Autodesk Inventor part; units mm, degrees
ref_plane "YZ Plane" through (0, 0, 0) normal (1, 0, 0) x (0, 1, 0)
ref_plane "XZ Plane" through (0, 0, 0) normal (0, 1, 0) x (-1, 0, 0)
ref_plane "XY Plane" through (0, 0, 0) normal (0, 0, 1) x (1, 0, 0)
sketch "スケッチ1" plane through (0, 0, 0) normal (0, 0, 1) x (1, 0, 0)
  line L0 (0, 0) -> (10, 0)
  line L1 (10, 0) -> (10, 15)
  line L2 (10, 15) -> (0, 15)
  line L3 (0, 15) -> (0, 0)
  circle A0 centre (5, 15) radius 8.5
  point P0 (0, 8.1261)
  point P1 (10, 8.1261)
  dimension "d0" = 15
  dimension "d1" = 17
  dimension "d27" = 10
  dimension "d28" = 5
extrude "押し出し1" add sketch "スケッチ1" along normal blind 9
sketch "スケッチ2" plane through (0, 0, 9) normal (0, 0, 1) x (1, 0, 0)
  arc A0 (10, 8.1261) -> (0, 8.1261) centre (5, 15) ccw
  point P0 (0, 0)
hole "穴1" at (5, 15, 9) direction (0, 0, -1) diameter 8.3 end through all
sketch "スケッチ3" plane through (0, 0, 9) normal (0, 0, 1) x (1, 0, 0)
  line L0 (0, 0) -> (10, 0)
  line L1 (4.5, 0) -> (5.5, 0)
  line L2 (5.5, 0) -> (5.5, 15)
  line L3 (5.5, 15) -> (4.5, 15)
  line L4 (4.5, 15) -> (4.5, 0)
  line L5 (0, 8.1261) -> (0, 0)
  circle A0 centre (5, 15) radius 4.15
  point P0 (5, 0)
  point P1 (5, 0)
  dimension "d14" = 1
extrude "押し出し2" cut sketch "スケッチ3" against normal up to surface (9 mm away) contours L4 A0 L2 L0 | L4 L3 L2 A0 picked at (4.9443, 13.6178)
sketch "スケッチ4" plane through (10, 0, 0) normal (1, 0, 0) x (0, 0, -1)
  circle A0 centre (-4.5, 4) radius 1.5
  line L0 (0, 0) -> (-9, 0)
  line L1 (0, 0) -> (0, 8.1261)
  line L2 (-4.5, 0) -> (-4.5, 10)
  point P0 (0, 10)
  dimension "d17" = 4
  dimension "d19" = 3
hole "穴2" at (10, 4, 4.5) direction (-1, 0, 0) diameter 4.4 end through all
sketch "スケッチ7" plane through (10, 0, 0) normal (1, 0, 0) x (0, 0, -1)
  circle A0 centre (-4.5, 4) radius 2.2
  line L0 (-4.5, 8.1569) -> (-0.9, 6.0785)
  line L1 (-0.9, 6.0785) -> (-0.9, 1.9215)
  line L2 (-0.9, 1.9215) -> (-4.5, -0.1569)
  line L3 (-4.5, -0.1569) -> (-8.1, 1.9215)
  line L4 (-8.1, 1.9215) -> (-8.1, 6.0785)
  line L5 (-8.1, 6.0785) -> (-4.5, 8.1569)
  line L6 (-9, 10.8802) -> (-9, 0)
  line L7 (0, 0) -> (0, 8.1261)
  line L8 (-9, 10.8802) -> (0, 10.8802)
  line L9 (0, 10.8802) -> (0, 4.0631)
  line L10 (0, 4.0631) -> (-9, 4.0631)
  line L11 (-9, 4.0631) -> (-9, 10.8802)
  point P0 (-4.5, 4)
  point P1 (-0.9, 4.0631)
  point P2 (-8.1, 4.0631)
  dimension "d35" = 7.2
extrude "押し出し5" add sketch "スケッチ7" along normal blind 2 contours L1 L0 L5 L4 L10 L6 L8 L9 L7
chamfer "面取り1" distance 2 angle 45 2 edges at (10, 4.0631, 8.55) (10, 4.0631, 0.45)
equation "\"d28\" = 0.5 * d27"
properties part number "軸止め" material "ABS プラスチック"
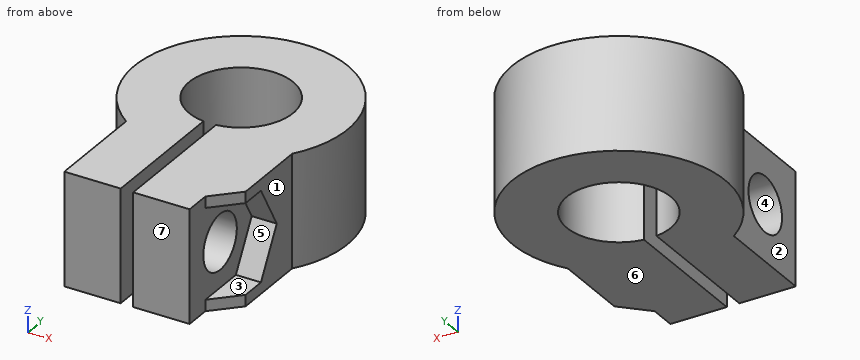
Source: CAD feature listing. Evaluate the final solid. Frame: model axes, mm. Face numbers are marked on the shaded views. A direction names the side the tool comes from. Give positions to 0.01 mm unless a question says otherwise; leave off trailing zeros. Loops run counter-clockwise (first coordinate to the right, second up) from the corner with the lowest first, then second, coordinate; pieces in that order, holes last. Notation, with made-up numbers: M 66,26.25 L 105,26.25 A21 ccw 105,42.25 Z; hole C 33,-17 d1. An arc over 180 degrees is marked long. Put each result on its own line as item: value.
Q1. Section D-D (y = 7.75). Return the cut outline in (x, z).
Response values:
outline: M 0,0 L 4.5,0 L 4.5,9 L 0,9 Z; M 5.5,0 L 12,0 L 12,3.8 L 10,3.8 L 10,5.2 L 12,5.2 L 12,9 L 5.5,9 Z
Q2. Line query: probe 1 along X at (y, z) = (3, 1); probe 2 along Y at (x, z) = (2, 5); probe 3 along Y at (x, z) = (1.9, 4.5). Output: solid intervals per line, ascending. Write a range as [from, to].
Response values:
probe 1: x = [0, 4.5], [5.5, 10]
probe 2: y = [0, 1.86], [6.14, 12.13], [17.87, 22.95]
probe 3: y = [0, 1.8], [6.2, 12.24], [17.76, 22.91]
Q3. Section A-A (y = 15). Return the cut outline in (x, z), and give its area (3 significant figures).
Response values:
outline: M -3.5,0 L 0.85,0 L 0.85,9 L -3.5,9 Z; M 9.15,0 L 13.5,0 L 13.5,9 L 9.15,9 Z
area: 78.3 mm²
Q4. Mould query, pull axis Z, two halves, no side actions, for the marked faces 4, 5, 6 and 7. Classes: released by +Z, released by -Z, zero draft, split by the parting line, or undercut.
Response values:
face 4: undercut
face 5: undercut
face 6: released by -Z
face 7: zero draft
Q5. Section B-B (x = 4.25). Return the cut outline in (y, z).
Response values:
outline: M 0,0 L 10.92,0 L 10.92,9 L 0,9 Z; M 19.08,0 L 23.47,0 L 23.47,9 L 19.08,9 Z; hole C 4,4.5 d4.4
Q6. Reachability of the marked faces 1, 2 and 3 from +Z, -Z, +X, -X, +Y, -Y: full face, straight path, thin tool, end or side. Return the list, or none.
Response values:
face 1: +Z, -Z, +X, -Y
face 2: +Z, -Z, -X, -Y
face 3: +X, -Y
Q7. Section C-C (x = 8.75). Return the cut outline in (y, z).
Response values:
outline: M 0,0 L 13.22,0 L 13.22,9 L 0,9 Z; M 16.78,0 L 22.63,0 L 22.63,9 L 16.78,9 Z; hole C 4,4.5 d4.4
Q8. Pin query (flat end, axial travel): P1, Ø4.5, axis at y = 3.5, z = 5.5, coming from the -X side; P2, Ø9.5, axis at x = 5, y = 15, coming from the -Z side; P3, Ø5, axis at y = 8, z = 2.5, coming from the +X side; P4, Ø5, axis at x = 4.5, y = 16, coming from the +Z side. Return the tip coordinate at first contact, or that it passes through.
Response values:
P1: stops at x = 0
P2: stops at z = 0
P3: stops at x = 12.21
P4: passes through
